Geometry: final body of the model. Coordinates: model frame, mm. Give positions to 0.01 mm unless a question says otherwise; leave off trailing zeros. Loops run counter-clockwise (first coordinate to the right, second up) from the corner with the lowest first, then second, coordinate; pieces in that order, holes last.
1. Section C-C, the plane y = 44.5. Output: boundary loops of the cut face in (x, z).
2. First-contact query: P1, Ø0.9, axis at x = 36.5, z = 1.5, coming from the -Y side. Flat tip, straight axial feed; report the tip coordinate or a pass-through.
3. Section B-B, the plane x = 8. Output: boundary loops of the cut face in (y, z).
4. Section A-A, the plane z = 1.75. Output: boundary loops of the cut face in (x, y), then the cut area to 3 significant figures.
5. Material intervals for line 1 along Y through (x, z) = (3, 2.7); line 2 along X through (y, z) = (57, 1.5); line 3 along X through (y, z) = (3, 1.45), sorted ascending.
from build123d import *

# Parameters (mm, degrees)
F0_R     = 0.7
F1_DEPTH = 3


with BuildPart() as f1:
    # F0 (on Top) → F1 (new body)
    with BuildSketch(Plane.XY):
        with BuildLine():
            Line((0, 75), (0, 0))
            Line((0, 0), (6, 0))
            Line((6, 0), (6, 69))
            ThreePointArc((6, 69), (7.464466, 72.535534), (11, 74))
            Line((11, 74), (19.39934, 74))
            Line((19.39934, 74), (46, 74))
            Line((46, 74), (46, 80))
            Line((46, 80), (6, 80))
            Line((6, 80), (5, 80))
            ThreePointArc((5, 80), (1.464466, 78.535534), (0, 75))
        make_face()
        with Locations((3, 2.840546)):
            Circle(F0_R, mode=Mode.SUBTRACT)
        with Locations((3, 16.040546)):
            Circle(F0_R, mode=Mode.SUBTRACT)
    extrude(amount=F1_DEPTH)


solid = f1.part
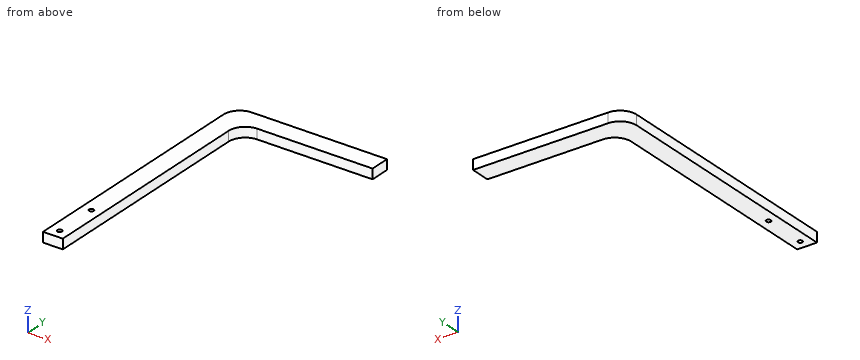
Answers below:
1. outline: (0, 0) - (6, 0) - (6, 3) - (0, 3) - close
2. P1: stops at y = 74
3. outline: (73, 0) - (80, 0) - (80, 3) - (73, 3) - close
4. outline: (0, 0) - (6, 0) - (6, 69) arc R5 cw to (11, 74) - (46, 74) - (46, 80) - (5, 80) arc R5 ccw to (0, 75) - close; hole circle Ø1.4 at (3, 2.84); hole circle Ø1.4 at (3, 16.04)
4. area: 717 mm2
5. line 1: y = 0 to 2.14, 3.54 to 15.34, 16.74 to 79.58
5. line 2: x = 0 to 6
5. line 3: x = 0 to 2.32, 3.68 to 6
